from build123d import *

# Parameters (mm, degrees)
SKETCH_1_R          = 2.5
EXTRUDE_1_DEPTH     = 180
SKETCH_2_R          = 82.250528809
CUT_EXTRUDE_1_DEPTH = 10
SKETCH_3_R          = 47.359827943
CUT_EXTRUDE_2_DEPTH = 200


with BuildPart() as part:
    # 草图1 → 凸台-拉伸1 (new, symmetric)
    with BuildSketch(Plane(origin=(0, 0, 0), x_dir=(1, 0, 0), z_dir=(0, 1, 0))):
        Polygon((-15, -3.15), (-12.5, -3.15), (-12.5, -5.15), (-7, -5.15), (-7, -3.15), (-4.5, -3.15), (-4.5, 3.15), (-7, 3.15), (-7, 5.15), (-12.5, 5.15), (-12.5, 3.15), (-15, 3.15), (-15, 15), (-3.15, 15), (-3.15, 12.5), (-5.15, 12.5), (-5.15, 7), (-3.15, 7), (-3.15, 4.5), (3.15, 4.5), (3.15, 7), (5.15, 7), (5.15, 12.5), (3.15, 12.5), (3.15, 15), (15, 15), (15, 3.15), (12.5, 3.15), (12.5, 5.15), (7, 5.15), (7, 3.15), (4.5, 3.15), (4.5, -3.15), (7, -3.15), (7, -5.15), (12.5, -5.15), (12.5, -3.15), (15, -3.15), (15, -15), (3.15, -15), (3.15, -12.5), (5.15, -12.5), (5.15, -7), (3.15, -7), (3.15, -4.5), (-3.15, -4.5), (-3.15, -7), (-5.15, -7), (-5.15, -12.5), (-3.15, -12.5), (-3.15, -15), (-15, -15), align=None)
        with Locations(Location((-9.75, -9.75, 0), (0, 0, 90))):
            Circle(SKETCH_1_R, mode=Mode.SUBTRACT)
        with Locations(Location((-9.75, 9.75, 0), (0, 0, 90))):
            Circle(SKETCH_1_R, mode=Mode.SUBTRACT)
        with Locations(Location((9.75, 9.75, 0), (0, 0, 90))):
            Circle(SKETCH_1_R, mode=Mode.SUBTRACT)
        with Locations(Location((9.75, -9.75, 0), (0, 0, 90))):
            Circle(SKETCH_1_R, mode=Mode.SUBTRACT)
    extrude(amount=EXTRUDE_1_DEPTH, both=True)

    # 草图2 → 切除-拉伸1 (cut)
    with BuildSketch(Plane(origin=(0, 180, 0), x_dir=(1, 0, 0), z_dir=(0, 1, 0))):
        Circle(SKETCH_2_R)
    extrude(amount=-CUT_EXTRUDE_1_DEPTH, mode=Mode.SUBTRACT)

    # 草图3 → 切除-拉伸2 (cut)
    with BuildSketch(Plane.XZ.offset(180)):
        with Locations((0.216432031, -1.772037256)):
            Circle(SKETCH_3_R)
    extrude(amount=-CUT_EXTRUDE_2_DEPTH, mode=Mode.SUBTRACT)


solid = part.part
Build history of the part. All positions in model axes, mm. A direction names the side the tool comes from. Give positions to 0.01 mm unless a question says otherwise; leave off trailing zeros. Write each loop counter-clockwise with the first axis right and the second up, starting at its lowest first coordinate (ties: lowest second). Pieces come first, ordered by that corner, then holes. Notation, with made-up numbers: (20, 3) - (24, 3) arc R18 ccw to (24, 31) - close; hole circle Ø6 at (-25.75, 70.5). An arc over 180 degrees is marked (long way). Use one line per item in the form item = value. Start each with the question number.
1. Drop a flat-ended pin along its axis: pin 1 Ø3 at (y, z) = (110, -1.5) entering from -X. Give the stop position or say it passes through.
2. Probe line 1 (X direction, y = 123, z = -9.75); line 2 (Z direction, x = 5, y = 94.5); line 3 (X direction, y = 114.5, z = -7.75). List the from-to ranges inside material, lowest first. Write a range as [from, to].
3. 3-axis set-ups, long thin cutter, end or side, ignore diameter. For faces 1 (the face through (0, 96, 4.5)), 2 (the face through (-5.15, 96, -10)), 3 (the face through (14, 96, 3.15)), 4 (the face through (-3.15, 96, -6)), 5 (the face through (-14, 96, -3.15)): which of +Z, -Z, +X, -X, +Y, -Y reach the whole face in a straight line?
4. Band-saw the part on C-C on y = 159. Count the separate pieces of the cut face and the enclosed holes in it, plus the area to 3 significant figures.
5. Band-saw the part on D-D on x = 1.5. Write the cut outline in (y, z).
6. Band-saw the part on B-B on z = -9.75. Write the cut outline in (x, y), plus the area to 4 significant figures.
7. Band-saw the part on A-A on x = -9.75. Write the cut outline in (y, z).
Conclusion:
q1.pin_1 = -4.5
q2.line_1 = [-15, -12.25], [-7.25, -5.15], [5.15, 7.25], [12.25, 15]
q2.line_2 = [-15, -12.5], [-7, -3.15], [3.15, 7], [12.5, 15]
q2.line_3 = [-15, -11.25], [-8.25, -5.15], [5.15, 8.25], [11.25, 15]
q3.face_1 = +Z, +Y, -Y
q3.face_2 = +Y, -Y
q3.face_3 = +X, +Y, -Y
q3.face_4 = -Z, +Y, -Y
q3.face_5 = -X, +Y, -Y
q4.separate_pieces = 1
q4.enclosed_holes = 4
q4.area = 469 mm²
q5.outline = (20, -4.5) - (170, -4.5) - (170, 4.5) - (20, 4.5) - close
q6.outline = (-15, 20) - (-12.25, 20) - (-12.25, 170) - (-15, 170) - close; (-7.25, 20) - (-5.15, 20) - (-5.15, 170) - (-7.25, 170) - close; (5.15, 20) - (7.25, 20) - (7.25, 170) - (5.15, 170) - close; (12.25, 20) - (15, 20) - (15, 170) - (12.25, 170) - close
q6.area = 1,455 mm²
q7.outline = (20, -15) - (170, -15) - (170, -12.25) - (20, -12.25) - close; (20, -7.25) - (170, -7.25) - (170, -5.15) - (20, -5.15) - close; (20, 5.15) - (170, 5.15) - (170, 7.25) - (20, 7.25) - close; (20, 12.25) - (170, 12.25) - (170, 15) - (20, 15) - close
